For this review, take the finished solid that the model builds, in its own axes (mm). Face numbers are marked on the shaded views. A direction names the side the tool comes from. Coordinates: 2 decimals unless noted, no trailing zeros. Loops run counter-clockwise (first coordinate to the right, second up) from the corner with the lowest first, then second, coordinate; pieces in that order, holes last. Notation, with made-up numbers: (85.25, 55.25) -> (134.25, 55.25) arc R22 ccw to (134.25, 93.25) -> close; hole circle Ø2 at (75.5, -35.75). An arc over 180 degrees is marked (long way). One line per item, written item: value.
from build123d import *

# Parameters (mm, degrees)
F1_DEPTH = 127
F2_T     = -10.16
F4_D     = 25.4
F4_DEPTH = 27.81203442
F5_W     = 30.5300801992
F5_H     = 70.8724632859
F6_DEPTH = 56.7313879728
F7_D     = 25.4
F7_DEPTH = 97.2380505333
F8_R     = 15.24
F9_R     = 5.08


with BuildPart() as f1:
    # F0 (on Front) → F1 (new body)
    with BuildSketch(Plane.XZ):
        with BuildLine():
            Line((-41.2577867825, 0), (-41.2577867825, -69.9788480997))
            Line((-41.2577867825, -69.9788480997), (42.0852601528, -69.9788480997))
            Line((42.0852601528, -69.9788480997), (42.0852601528, 0))
            ThreePointArc((42.0852601528, 0), (28.5956049165, 10.9886772048), (24.0628808213, 27.7867794006))
            Line((24.0628808213, 27.7867794006), (-23.52851646, 27.81103442))
            ThreePointArc((-23.52851646, 27.81103442), (-27.6884119308, 10.9062903381), (-41.2577867825, 0))
        make_face()
    extrude(amount=F1_DEPTH)

    # F2
    f2_openings = [f1.faces().sort_by_distance(p)[0] for p in [
        (0.418317, -127, -24.869702),
    ]]
    offset(amount=F2_T, openings=f2_openings)

    # F4 (through all, one way)
    with BuildSketch(Plane(origin=(0, 0, 0), x_dir=(1, 0, 0), z_dir=(0, 0, -1))):
        with Locations((0, 27.3138843477)):
            Circle(F4_D / 2)
    extrude(amount=-F4_DEPTH, mode=Mode.SUBTRACT)

    # F5 (on Front) → F6 (join)
    with BuildSketch(Plane.XZ):
        with Locations((0, 61.8008188903)):
            Rectangle(F5_W, F5_H)
    extrude(amount=F6_DEPTH)

    # F7 (through all, one way)
    with BuildSketch(Plane(origin=(0, 0, 0), x_dir=(1, 0, 0), z_dir=(0, 0, -1))):
        with Locations((0, 27.3138843477)):
            Circle(F7_D / 2)
    extrude(amount=-F7_DEPTH, mode=Mode.SUBTRACT)

    # F8
    f8_edges = [f1.edges().sort_by_distance(p)[0] for p in [
        (15.26504, 0, 62.514157),
        (-15.26504, 0, 62.521937),
        (15.26504, -56.731388, 62.514157),
        (-15.26504, -56.731388, 62.521937),
    ]]
    fillet(f8_edges, radius=F8_R)

    # F9
    f9_edges = [f1.edges().sort_by_distance(p)[0] for p in [
        (42.08526, -63.5, 0),
        (24.062881, -63.5, 27.786779),
        (-23.528516, -63.5, 27.811034),
        (-41.257787, -63.5, 0),
        (-27.688412, 0, 10.90629),
        (-27.688412, -127, 10.90629),
    ]]
    fillet(f9_edges, radius=F9_R)


solid = f1.part
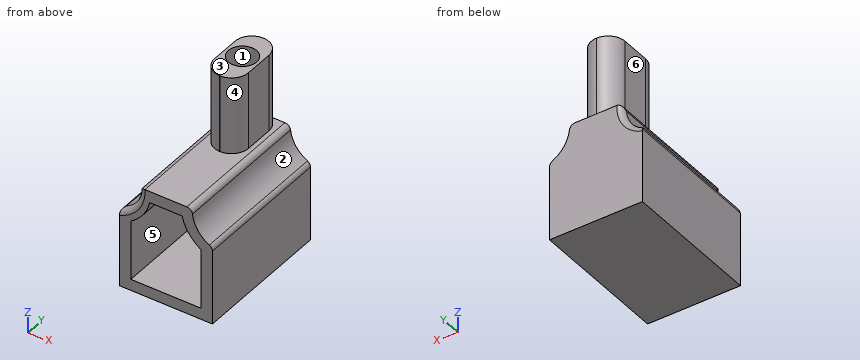
1. To check wall thickness, follow probe 1 along Z at (x, y) = (-12.5, -15.5); probe 2 along Y at (x, z) = (0, 37.5); probe 3 along Z at (x, y) = (1, -106). State the ranges of each line that lie inside material, in increasing order. Write a range as from..to.
Return value:
probe 1: z = -69.98..-59.82, 17.65..97.24
probe 2: y = -56.73..-40.01, -14.61..0
probe 3: z = -69.98..-59.82, 17.64..27.8
2. The part is to be moulded in two halves that separate along X. For the marked faces 1, 2 and 3, say which applies: pulls with the +X half, pulls with the -X half, needs draft (parallel to the pull), parting line crosses it, or undercut.
Return value:
face 1: undercut
face 2: pulls with the +X half
face 3: needs draft
3. Insertion check: pin 1 Ø13 at (y, z) = (-25.5, 71.5) entering from +X; pin 2 Ø1.5 at (y, z) = (-74.5, 11.5) entering from +X; pin 3 Ø21 at (y, z) = (-26.5, 60) entering from -X. Each pin has a flat end and moves straight along its axis. Give the tip position at first contact, or say it passes through.
Return value:
pin 1: stops at x = 15.27
pin 2: stops at x = 28.75
pin 3: stops at x = -15.27
4. Take a section at C-C, the plane x = -8. Give the boundary of the cut face in (y, z), and give its area (3 significant figures).
Return value:
outline: (-127, -69.98) -> (0, -69.98) -> (0, 27.8) -> (-2.25, 27.8) -> (-2.25, 97.24) -> (-17.45, 97.24) -> (-17.45, 17.64) -> (-10.16, 17.64) -> (-10.16, -59.82) -> (-127, -59.82) -> close; (-127, 17.64) -> (-37.18, 17.64) -> (-37.18, 97.24) -> (-54.48, 97.24) -> (-54.48, 27.8) -> (-127, 27.8) -> close
area: 5,420 mm2
5. Take a section at A-A, the plane z = -10.5. Give the boundary of the cut face in (x, y), and give its area (3 significant figures).
Return value:
outline: (-41.26, -127) -> (-31.1, -127) -> (-31.1, -10.16) -> (31.93, -10.16) -> (31.93, -127) -> (42.09, -127) -> (42.09, 0) -> (-41.26, 0) -> close
area: 3,220 mm2
6. Take a section at B-B, the plane y = -104. Give the boundary of the cut face in (x, z).
Return value:
outline: (-41.26, -69.98) -> (42.09, -69.98) -> (42.09, -3.27) arc R5.08 ccw to (39.34, 1.24) arc R28.36 cw to (24.2, 23.27) arc R5.08 ccw to (19.16, 27.79) -> (-18.47, 27.81) arc R5.08 ccw to (-23.53, 23.17) arc R27.16 cw to (-38.45, 1.21) arc R5.08 ccw to (-41.26, -3.33) -> close; hole (-31.1, -59.82) -> (31.93, -59.82) -> (31.93, -6.21) arc R38.52 cw to (14.89, 17.63) -> (-14.11, 17.65) arc R37.32 cw to (-31.1, -6.32) -> close
7. Take a section at D-D, the plane z = 65.5. Give the boundary of the cut face in (x, y), and give its area (3 significant figures).
Return value:
outline: (-15.27, -41.49) arc R15.24 ccw to (-0.03, -56.73) -> (0.03, -56.73) arc R15.24 ccw to (15.27, -41.49) -> (15.27, -15.24) arc R15.24 ccw to (0.03, 0) -> (-0.03, 0) arc R15.24 ccw to (-15.27, -15.24) -> close; hole circle Ø25.4 at (0, -27.31)
area: 1,030 mm2
8. For the marked faces 4, 5 and 6, list the 3-axis set-ups (+Z, -Z, +X, -X, +Y, -Y) from which the entire face can be reached by the end or side of a thin tool; tool diameter is ignored.
Return value:
face 4: +Z, +X, -Y
face 5: -Y
face 6: +Z, -X, +Y, -Y
